from build123d import *

# Parameters (mm, degrees)
SKETCH1_W           = 558.8
SKETCH1_H           = 889
BOSS_EXTRUDE1_DEPTH = 762
BOSS_EXTRUDE2_DEPTH = 558.8
SKETCH4_W           = 533.4
SKETCH4_H           = 127
CUT_EXTRUDE1_DEPTH  = 763
SKETCH5_W           = 533.4
SKETCH5_H           = 723.9
CUT_EXTRUDE3_DEPTH  = 755.142
SKETCH6_W           = 533.4
SKETCH6_H           = 889
CUT_EXTRUDE4_DEPTH  = 10.16
SKETCH7_R           = 38.1
CUT_EXTRUDE5_DEPTH  = 559.8
CUT_EXTRUDE6_DEPTH  = 533.908
CUT_EXTRUDE7_REACH  = 764
SKETCH12_W          = 533.4
SKETCH12_H          = 12.7
SKETCH13_R          = 2.5
SKETCH13_R_2        = 12.7
BOSS_EXTRUDE3_DEPTH = 6.35
SKETCH14_R          = 12.7
SKETCH14_R_2        = 2.5
CUT_EXTRUDE8_DEPTH  = 6.35
SKETCH15_R          = 12.7
CUT_EXTRUDE9_DEPTH  = 6.35


with BuildPart() as part:
    # Sketch1 → Boss-Extrude1 (new body)
    with BuildSketch(Plane.XY):
        with Locations((279.4, 444.5)):
            Rectangle(SKETCH1_W, SKETCH1_H)
    extrude(amount=BOSS_EXTRUDE1_DEPTH)

    # Sketch3 → Boss-Extrude2 (add)
    with BuildSketch(Plane(origin=(558.8, 0, 0), x_dir=(0, 0, -1), z_dir=(1, 0, 0))):
        Polygon((0, 889), (0, 1270), (-762, 889), align=None)
    extrude(amount=-BOSS_EXTRUDE2_DEPTH)

    # Sketch4 → Cut-Extrude1 (cut, through all)
    with BuildSketch(Plane.XY.offset(762)):
        with Locations((279.4, 76.2)):
            Rectangle(SKETCH4_W, SKETCH4_H)
    extrude(amount=-CUT_EXTRUDE1_DEPTH, mode=Mode.SUBTRACT)

    # Sketch5 → Cut-Extrude3 (cut)
    with BuildSketch(Plane.XY.offset(762)):
        with Locations((279.4, 514.35)):
            Rectangle(SKETCH5_W, SKETCH5_H)
    extrude(amount=-CUT_EXTRUDE3_DEPTH, mode=Mode.SUBTRACT)

    # Sketch6 → Cut-Extrude4 (cut)
    with BuildSketch(Plane(origin=(0, 0, 0), x_dir=(-1, 0, 0), z_dir=(0, 0, -1))):
        with Locations((-279.4, 800.1)):
            Rectangle(SKETCH6_W, SKETCH6_H)
    extrude(amount=-CUT_EXTRUDE4_DEPTH, mode=Mode.SUBTRACT)

    # Sketch7 → Cut-Extrude5 (cut, through all)
    with BuildSketch(Plane.ZY):
        with Locations((123.444, 712.216)):
            Circle(SKETCH7_R)
    extrude(amount=-CUT_EXTRUDE5_DEPTH, mode=Mode.SUBTRACT)

    # Sketch11 → Cut-Extrude6 (cut)
    with BuildSketch(Plane.ZY.offset(-546.1)):
        Polygon((0, 880.877149752), (0, 1247.656728703), (749.847637181, 880.877149752), (749.847637181, 851.37553613), (0, 851.37553613), align=None)
    extrude(amount=CUT_EXTRUDE6_DEPTH, mode=Mode.SUBTRACT)

    # Sketch12 → Cut-Extrude7 (cut, up to next)
    with BuildSketch(Plane.XY.offset(762), mode=Mode.PRIVATE) as cut_extrude7_sk1:
        with Locations((279.4, 146.05)):
            Rectangle(SKETCH12_W, SKETCH12_H)
    cut_extrude7_tool1 = extrude(cut_extrude7_sk1.sketch, amount=-CUT_EXTRUDE7_REACH, mode=Mode.PRIVATE) & part.part
    add(cut_extrude7_tool1.solids().sort_by_distance((279.4, 146.05, 762))[0], mode=Mode.SUBTRACT)

    # Sketch13 → Boss-Extrude3 (add)
    with BuildSketch(Plane.ZY):
        with Locations((45, 955.20656175)):
            Circle(SKETCH13_R)
        with Locations((25, 955.20656175)):
            Circle(SKETCH13_R)
        with Locations((35, 935.20656175)):
            Circle(SKETCH13_R)
        with Locations((15, 935.20656175)):
            Circle(SKETCH13_R)
        with Locations((740.165987986, 807.854465699)):
            Circle(SKETCH13_R_2)
        with Locations((35, 314.79343825)):
            Circle(SKETCH13_R)
        with Locations((45, 334.79343825)):
            Circle(SKETCH13_R)
        with Locations((25, 334.79343825)):
            Circle(SKETCH13_R)
        with Locations((15, 314.79343825)):
            Circle(SKETCH13_R)
    extrude(amount=BOSS_EXTRUDE3_DEPTH)

    # Sketch14 → Cut-Extrude8 (cut)
    with BuildSketch(Plane(origin=(558.8, 0, 0), x_dir=(0, 0, -1), z_dir=(1, 0, 0))):
        with Locations((-87.309700123, 1127.19181172)):
            Circle(SKETCH14_R)
        with Locations((-740.165987986, 807.854465699)):
            Circle(SKETCH14_R)
        with Locations((-25, 935.20656175)):
            Circle(SKETCH14_R_2)
        with Locations((-45, 935.20656175)):
            Circle(SKETCH14_R_2)
        with Locations((-35, 955.20656175)):
            Circle(SKETCH14_R_2)
        with Locations((-15, 955.20656175)):
            Circle(SKETCH14_R_2)
        with Locations((-25, 314.79343825)):
            Circle(SKETCH14_R_2)
        with Locations((-45, 314.79343825)):
            Circle(SKETCH14_R_2)
        with Locations((-35, 334.79343825)):
            Circle(SKETCH14_R_2)
        with Locations((-15, 334.79343825)):
            Circle(SKETCH14_R_2)
    extrude(amount=-CUT_EXTRUDE8_DEPTH, mode=Mode.SUBTRACT)

    # Sketch15 → Cut-Extrude9 (cut)
    with BuildSketch(Plane.ZY):
        with Locations((87.309700123, 1127.19181172)):
            Circle(SKETCH15_R)
    extrude(amount=-CUT_EXTRUDE9_DEPTH, mode=Mode.SUBTRACT)


solid = part.part
Could you check a few things on this model? Use its own coordinates, in mm. A direction names the side the tool comes from. Give positions to 0.01 mm unless a question says otherwise; leave off trailing zeros. Loops run counter-clockwise (first coordinate to the right, second up) from the corner with the lowest first, then second, coordinate; pieces in that order, holes last. Notation, with made-up numbers: (43.5, 14) -> (91.5, 14) arc R14 ccw to (91.5, 31) -> close; hole circle Ø2 at (34, -18.5). An arc over 180 degrees is marked (long way). Return JSON: item names as keys, results as strings.
Item 1: Which directions (+Z, -Z, +X, -X, +Y, -Y) give clear straight access to the entire face, cutting with the end or side of a thin tool? Please do faces 1 (the flat face through (12.192, 964, 297)), 2 (the flat face through (12.7, 438, 386)), 3 (the cylindrical face through (-3.131, 820.446, 738.513)).
Geometry results:
{"face 1": "-Z", "face 2": "+Z", "face 3": "-X"}
Item 2: If we section it at A-A on x = 139.5: List the corners of the cut face in (y, z) for me.
Geometry results:
{"outline": "(0, 0) -> (12.7, 0) -> (12.7, 762) -> (0, 762) -> close; (152.4, 0) -> (355.6, 0) -> (355.6, 6.86) -> (152.4, 6.86) -> close; (876.3, 749.85) -> (880.88, 749.85) -> (1242.69, 10.16) -> (1244.6, 10.16) -> (1244.6, 6.25) -> (1247.66, 0) -> (1270, 0) -> (889, 762) -> (876.3, 762) -> close"}
Item 3: If we section it at C-C on z = 693: List the corners of the cut face in (x, y) for me, plus the area to 3 significant figures.
Geometry results:
{"outline": "(0, 0) -> (558.8, 0) -> (558.8, 923.5) -> (0, 923.5) -> close; hole (12.19, 851.38) -> (12.7, 851.38) -> (12.7, 12.7) -> (546.1, 12.7) -> (546.1, 908.68) -> (12.19, 908.68) -> close", "area": "38,100 mm²"}
Item 4: If we section it at B-B on y = 283: List the corners of the cut face in (x, z) for me.
Geometry results:
{"outline": "(0, 0) -> (558.8, 0) -> (558.8, 762) -> (546.1, 762) -> (546.1, 6.86) -> (12.7, 6.86) -> (12.7, 762) -> (0, 762) -> close"}
Item 5: I need wall thicknesses on L1, parallel to Y at x = 554, z = 45; L2, parallel to X at y = 601.5, z = 624.5; L3, parallel to X at y = 1028.5, z = 197. Which ranges of each line are inside material? Lowest first, please. Write a range as from..to.
Geometry results:
{"L1": "y = 0..312.29, 317.29..932.71, 937.71..1247.5", "L2": "x = 0..12.7, 546.1..558.8", "L3": "x = 0..12.19, 546.1..558.8"}
Item 6: I'm going to push flat-ended pins straight in: pin 1 (2 mm diameter, centred on x = 409, z = 231, fed in from -Y); pin 2 (9 mm diameter, centred on x = 407.5, y = 873.5, fed in from -Z); pin 3 (7.5 mm diameter, centred on y = 1127, z = 81, fed in from +X); pin 4 (2 mm diameter, centred on x = 270.5, y = 1243.5, fed in from -Z). Where does each tip first touch, or does it pass through?
Geometry results:
{"pin 1": "stops at y = 0", "pin 2": "stops at z = 749.85", "pin 3": "stops at x = 552.45", "pin 4": "stops at z = 10.16"}
Item 7: We'd pull the mould along Z, two halves only. Please class faces 4 (the flat face through (552.45, 808, 740)), 5 (the flat face through (558.8, 503, 386)), 6 (the flat face through (343, 350, 0)): +Z half, -Z half, draft (parallel to the pull), parting line (faces both ways), or undercut.
Geometry results:
{"face 4": "undercut", "face 5": "draft", "face 6": "-Z half"}
Item 8: If we section it at D-D on z = 283: List the corners of the cut face in (x, y) for me, plus the area to 3 significant figures.
Geometry results:
{"outline": "(0, 0) -> (558.8, 0) -> (558.8, 1128.5) -> (0, 1128.5) -> close; hole (12.19, 851.38) -> (12.7, 851.38) -> (12.7, 12.7) -> (546.1, 12.7) -> (546.1, 1109.23) -> (12.19, 1109.23) -> close", "area": "45,600 mm²"}
